from build123d import *

# Parameters (mm, degrees)
F0_W     = 36
F0_H     = 96
F1_DEPTH = 10
F2_W     = 48
F2_H     = 96
F3_DEPTH = 16
F4_W     = 48
F4_H     = 16
F5_DEPTH = 10
F6_W     = 19
F6_H     = 16
F7_DEPTH = 10


with BuildPart() as f1:
    # F0 (on Top) → F1 (new body)
    with BuildSketch(Plane.XY):
        Rectangle(F0_W, F0_H)
    extrude(amount=F1_DEPTH)

    # F2 (on face) → F3 (join)
    with BuildSketch(Plane.XY.offset(10)):
        Rectangle(F2_W, F2_H)
    extrude(amount=F3_DEPTH)

    # F4 (on face) → F5 (join)
    with BuildSketch(Plane.XY.offset(26)):
        with Locations((0, -40)):
            Rectangle(F4_W, F4_H)
    extrude(amount=F5_DEPTH)

    # F6 (on face) → F7 (cut)
    with BuildSketch(Plane.XY.offset(36)):
        with Locations((-14.5, -40)):
            Rectangle(F6_W, F6_H)
        with Locations((14.5, -40)):
            Rectangle(F6_W, F6_H)
    extrude(amount=-F7_DEPTH, mode=Mode.SUBTRACT)


solid = f1.part
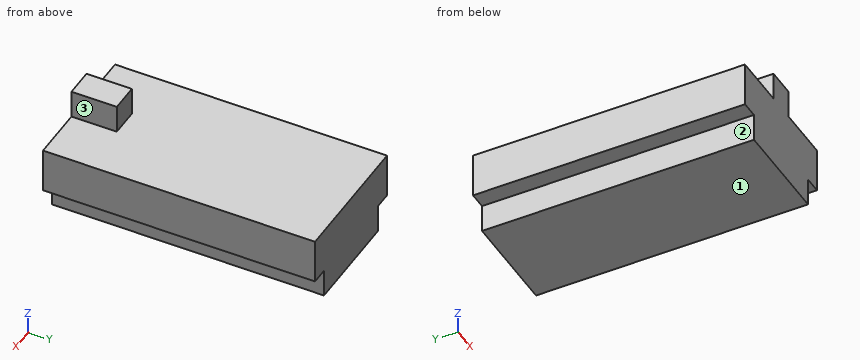
Verification items for the finished model (mm, model axes). Face numbers are marked on the shaded views. A direction names the side the tool comes from. Coordinates: 2 decimals unless noted, no trailing zeros. Write each loop counter-clockwise with the first axis right and the second up, starting at its lowest first coordinate (ties: lowest second). Pieces come first, ordered by that corner, then holes. Notation, with made-up numbers: (53.5, -7.5) - (78.5, -7.5) arc R26 ccw to (78.5, 23.5) - close; hole circle Ø9 at (4, -18.5). An arc over 180 degrees is marked (long way). Answer as a JSON object with one key per item and string values.
(1) Thickness scan on line 1 along Z through (x, y) = (-15.5, -12); line 2 along X through (y, z) = (7, 5); line 3 along Y through (x, z) = (1, 32). Record the ranges inside material, lowest first.
Report:
{"line 1": "0 to 26", "line 2": "-18 to 18", "line 3": "-48 to -32"}
(2) Cross-section at B-B on x = -2. Record the cut outline in (y, z), plus the area to 3 significant figures.
Report:
{"outline": "(-48, 0) - (48, 0) - (48, 26) - (-32, 26) - (-32, 36) - (-48, 36) - close", "area": "2,660 mm^2"}
(3) Cross-section at A-A on y = 28.5. Record the cut outline in (x, z), plus the area to 3 significant figures.
Report:
{"outline": "(-24, 10) - (-18, 10) - (-18, 0) - (18, 0) - (18, 10) - (24, 10) - (24, 26) - (-24, 26) - close", "area": "1,130 mm^2"}
(4) Gauge pin test, flat ends, axial feed: pin 1 Ø2 at (y, z) = (0.5, 8.5) entering from -X; pin 2 Ø5 at (x, y) = (-13, 30.5) entering from +Z; pin 3 Ø6 at (x, z) = (-18, 27) entering from +Y; pin 4 Ø3 at (x, y) = (-21, 0.5) entering from -Z. Record the tip position at first contact, or that the pin passes through.
Report:
{"pin 1": "x = -18", "pin 2": "z = 26", "pin 3": "y = 48", "pin 4": "z = 10"}
(5) Tool access check on the marked faces 1, 2 and 3. Record the directions out of +Z, -Z, +X, -X, +Y, -Y that give a thin tool (end or side, any length) a straight path to the whole face; none if there is none.
Report:
{"face 1": "-Z, +X, -X, +Y, -Y", "face 2": "-Z, -X, +Y, -Y", "face 3": "+Z, +X, +Y, -Y"}
(6) Cross-section at C-C on z = 29.5. Record the cut outline in (x, y).
Report:
{"outline": "(-5, -48) - (5, -48) - (5, -32) - (-5, -32) - close"}
(7) Cross-section at D-D on z = 6.5. Record the cut outline in (x, y), plus the area to 3 significant figures.
Report:
{"outline": "(-18, -48) - (18, -48) - (18, 48) - (-18, 48) - close", "area": "3,460 mm^2"}
